```python
from build123d import *

# Parameters (mm, degrees)
SKETCH_1_W               = 38
SKETCH_1_H               = 12
EXTRUDE_1_DEPTH          = 1.6
EXTRUDE_START            = 1.6
SKETCH_1_3_W             = 38
SKETCH_1_3_H             = 1
SKETCH_1_3_W_2           = 1.5
SKETCH_1_3_H_2           = 12
EXTRUDE_2_DEPTH          = 1.5
EXTRUDE_START_2          = 3.1
EXTRUDE_3_DEPTH          = 8.4
SKETCH_2_4_W             = 2.1
SKETCH_2_4_H             = 1.5
EXTRUDE_5_DEPTH          = 3.1
CUT_EXTRUDE_1_DEPTH      = 22.850629282
FILLET_1_R               = 3
EXTRUDE_4_REACH          = 28.771
SKETCH_3_R               = 1.45
CUT_EXTRUDE_2_DEPTH      = 27.771253239
CUT_EXTRUDE_2_DEPTH_BACK = 27.771253239
SKETCH_3_3_R             = 1.7
SKETCH_3_3_W             = 6.5
SKETCH_3_3_H             = 1.2
SKETCH_3_3_W_2           = 3.4
SKETCH_3_3_H_2           = 3.1
FILLET_2_R               = 2.8
FILLET_3_R               = 2.5
FILLET_4_R               = 1
FILLET_5_R               = 0.3
FILLET_6_R               = 2


with BuildPart() as part:
    # 草图1 → 凸台-拉伸1 (new body)
    with BuildSketch(Plane(origin=(0, 0, 0), x_dir=(1, 0, 0), z_dir=(0, 1, 0))):
        Rectangle(SKETCH_1_W, SKETCH_1_H)
    extrude(amount=EXTRUDE_1_DEPTH)

    # 草图1<3> → 凸台-拉伸2 (add)
    with BuildSketch(Plane(origin=(0, 0, 0), x_dir=(1, 0, 0), z_dir=(0, 1, 0)).offset(EXTRUDE_START)):
        with Locations((0, 4)):
            Rectangle(SKETCH_1_3_W, SKETCH_1_3_H)
        Rectangle(SKETCH_1_3_W, SKETCH_1_3_H)
        with Locations((0, -4)):
            Rectangle(SKETCH_1_3_W, SKETCH_1_3_H)
        with Locations((-11.75, 0)):
            Rectangle(SKETCH_1_3_W_2, SKETCH_1_3_H_2)
        with Locations((11.75, 0)):
            Rectangle(SKETCH_1_3_W_2, SKETCH_1_3_H_2)
    extrude(amount=EXTRUDE_2_DEPTH)

    # 草图2 → 凸台-拉伸3 (add)
    with BuildSketch(Plane(origin=(0, 0, 0), x_dir=(1, 0, 0), z_dir=(0, 1, 0)).offset(EXTRUDE_START_2)):
        Polygon((-3.3, 9.3), (-5.4, 9.3), (-5.4, -2.4), (-7.5, -2.4), (-7.5, -9.4), (-5.5, -9.4), (-5.5, -2.8), (-3.3, -2.8), align=None)
        Polygon((5.4, 9.3), (3.3, 9.3), (3.3, -2.8), (5.5, -2.8), (5.5, -9.4), (7.5, -9.4), (7.5, -2.4), (5.4, -2.4), align=None)
    extrude(amount=-EXTRUDE_3_DEPTH)

    # 草图2<4> → 凸台-拉伸5 (add)
    with BuildSketch(Plane(origin=(0, 0, 0), x_dir=(1, 0, 0), z_dir=(0, 1, 0))):
        with Locations((-6.45, 5.25)):
            Rectangle(SKETCH_2_4_W, SKETCH_2_4_H)
        with Locations((6.45, 5.25)):
            Rectangle(SKETCH_2_4_W, SKETCH_2_4_H)
    extrude(amount=EXTRUDE_5_DEPTH)

    # 草图2<3> → 切除-拉伸1 (cut, through all)
    with BuildSketch(Plane(origin=(0, 0, 0), x_dir=(1, 0, 0), z_dir=(0, 1, 0))):
        Polygon((0, -9.4), (0, -2.8), (-3.3, -2.8), (-5.4, -2.8), (-5.5, -2.8), (-5.5, -9.4), align=None)
        Polygon((3.3, -2.8), (0, -2.8), (0, -9.4), (5.5, -9.4), (5.5, -2.8), (5.4, -2.8), align=None)
    extrude(amount=CUT_EXTRUDE_1_DEPTH, mode=Mode.SUBTRACT)

    # 圆角1
    # the kernel refuses this fillet: 3 mm, written as the material it adds along each edge
    with BuildSketch(Plane(origin=(5.4, 7.154544011, 2.4), x_dir=(1, 0, 0), z_dir=(0, -1, 0))) as fillet_1_piece_1_section:
        with BuildLine():
            CenterArc((3, -2.861817604), FILLET_1_R, 107.457603124, 72.542396876)
            Line((0, -2.861817604), (0, 0))
            Line((0, 0), (2.1, 0))
        make_face()
    fillet_1_piece_1 = extrude(amount=12.454544011, mode=Mode.PRIVATE)
    fillet_1_piece_1 = split(fillet_1_piece_1, bisect_by=Plane(origin=(6.297598678, 1.6, 1.686657362), z_dir=(0, -1, 0)), keep=Keep.TOP, mode=Mode.PRIVATE)
    add(fillet_1_piece_1)
    with BuildSketch(Plane(origin=(-5.4, 0, 2.4), x_dir=(0, 0, -1), z_dir=(0, -1, 0))) as fillet_1_piece_2:
        with BuildLine():
            CenterArc((2.861817604, -3), FILLET_1_R, 90, 72.542396876)
            Line((0, -2.1), (0, 0))
            Line((0, 0), (2.861817604, 0))
        make_face()
    extrude(amount=5.3)

    # 草图3 → 凸台-拉伸4 (add, up to next)
    with BuildSketch(Plane(origin=(-5.5, 0, 0), x_dir=(0, 0, -1), z_dir=(1, 0, 0)), mode=Mode.PRIVATE) as extrude_4_sk1:
        with Locations((-7, -2.5)):
            Circle(SKETCH_3_R)
    extrude_4_tool1 = extrude(extrude_4_sk1.sketch, amount=EXTRUDE_4_REACH, mode=Mode.PRIVATE) - part.part
    add(extrude_4_tool1.solids().sort_by_distance((-5.5, -2.5, 7))[0])

    # 草图3<3> → 切除-拉伸2 (cut, two sides: drawn at the far end of the back side and taken through both)
    with BuildSketch(Plane(origin=(-5.5, 0, 0), x_dir=(0, 0, -1), z_dir=(1, 0, 0)).offset(-CUT_EXTRUDE_2_DEPTH_BACK)):
        with Locations((5.58, -2.5)):
            Circle(SKETCH_3_3_R)
        with Locations((6.05, -4.7)):
            Rectangle(SKETCH_3_3_W, SKETCH_3_3_H)
        with Locations((-7.7, 1.55)):
            Rectangle(SKETCH_3_3_W_2, SKETCH_3_3_H_2)
    extrude(amount=CUT_EXTRUDE_2_DEPTH + CUT_EXTRUDE_2_DEPTH_BACK, mode=Mode.SUBTRACT)

    # 圆角2
    # the kernel refuses this fillet: 2.8 mm, written as the material it takes off along each edge
    with BuildSketch(Plane(origin=(-1.5, 0, 9.4), x_dir=(0, 0, -1), z_dir=(1, 0, 0)), Plane(origin=(-14.5, 0, 9.4), x_dir=(0, 0, -1), z_dir=(1, 0, 0))) as fillet_2_piece_1:
        with BuildLine():
            CenterArc((FILLET_2_R, -FILLET_2_R), FILLET_2_R, 90, 90)
            Line((0, -FILLET_2_R), (0, 0))
            Line((0, 0), (FILLET_2_R, 0))
        make_face()
    extrude(amount=16, mode=Mode.SUBTRACT)
    with BuildSketch(Plane(origin=(-1.5, -5.3, 9.4), x_dir=(0, 0, -1), z_dir=(1, 0, 0)), Plane(origin=(-14.5, -5.3, 9.4), x_dir=(0, 0, -1), z_dir=(1, 0, 0))) as fillet_2_piece_2:
        with BuildLine():
            CenterArc((FILLET_2_R, FILLET_2_R), FILLET_2_R, 180, 90)
            Line((0, FILLET_2_R), (0, 0))
            Line((0, 0), (FILLET_2_R, 0))
        make_face()
    extrude(amount=16, mode=Mode.SUBTRACT)

    # 圆角3
    fillet_3_edges = [part.edges().sort_by_distance(p)[0] for p in [
        (-4.35, 3.1, -9.3),
        (4.35, 3.1, -9.3),
    ]]
    fillet(fillet_3_edges, radius=FILLET_3_R)

    # 圆角4
    fillet_4_edges = [part.edges().sort_by_distance(p)[0] for p in [
        (-4.35, -4.1, -9.3),
        (4.35, -4.1, -9.3),
    ]]
    fillet(fillet_4_edges, radius=FILLET_4_R)

    # 圆角5
    fillet_5_edges = [part.edges().sort_by_distance(p)[0] for p in [
        (-4.35, -4.1, -5.005543735),
        (4.35, -4.1, -5.005543735),
        (-4.35, -4.1, -6.154456265),
        (4.35, -4.1, -6.154456265),
    ]]
    fillet(fillet_5_edges, radius=FILLET_5_R)

    # 圆角6
    # the kernel refuses this fillet: 2 mm, written as the material it adds along each edge
    with BuildSketch(Plane(origin=(5.4, 3.1, 2.4), x_dir=(0, 0, -1), z_dir=(0, -1, 0))) as fillet_6_piece_1:
        with BuildLine():
            CenterArc((2, 1.997498436), FILLET_6_R, 180, 87.134016017)
            Line((0, 1.997498436), (-0.04, 1.997498436))
            Line((-0.04, 1.997498436), (-0.04, 0))
            Line((-0.04, 0), (0, -0.04))
            ThreePointArc((0, -0.04), (0.95, -0.04), (1.898, -0.039949969))
            Line((1.898, -0.039949969), (1.9, 0))
        make_face()
    extrude(amount=6.493746089)
    with BuildSketch(Plane(origin=(-5.4, 3.1, 2.4), x_dir=(-1, 0, 0), z_dir=(0, -1, 0))) as fillet_6_piece_2:
        with BuildLine():
            CenterArc((1.997498436, 2), FILLET_6_R, 182.865983983, 87.134016017)
            Line((0, 1.9), (-0.039949969, 1.898))
            ThreePointArc((-0.039949969, 1.898), (-0.04, 0.95), (-0.04, 0))
            Line((-0.04, 0), (0, -0.04))
            Line((0, -0.04), (1.997498436, -0.04))
            Line((1.997498436, -0.04), (1.997498436, 0))
        make_face()
    extrude(amount=6.493746089)


solid = part.part
```
Source: CAD feature listing. Evaluate the final solid. Frame: model axes, mm. A direction names the side the tool comes from. Give positions to 0.01 mm unless a question says otherwise; leave off trailing zeros. Order: outer loops, then holes, each group sorted by start corner. A loop starts at its lowest first (then second) coordinate and runs counter-clockwise, first axis right, second up.
(1) Material intervals for line 1 along Z through (x, y) = (-4, -2.5); line 2 along X through (y, z) = (-0.5, -5.5); line 3 along X through (y, z) = (-4, 5.5), sorted ascending.
(2) Contact query for flat-ended pins moving along their axis: P1, Ø1, axis at x = -2.5, z = -2, coming from the -Y side; P2, Ø1.6, axis at x = -10, y = 1, coming from the +Z side; P3, Ø1.6, axis at x = 8.5, y = 2.5, coming from the -Z side. Output: stop coordinate, or through.
(3) Section query D-D (x = -13). Return the cut outline in (y, z).
(4) Access query for faces 1 (the face through (12.5, 2, 2)), 2 (the face through (-9, 2, -4.5)), 3 (the face through (-11, 2, 5)), 4 (the face through (4, -4.1, -8)). Directions: +Z, -Z, +X, -X, +Y, -Y. A direction counts if a zero-diameter tool reaches every point of the face in a straight line with its end or side. Return the directions, or none.
(5) Section query C-C (z = -7.75). Return the cut outline in (x, y), plus the area to 3 significant figures.
(6) Section query B-B (y = -4.5). Return the cut outline in (x, z), plus the area to 3 significant figures.
(7) Section query A-A (x = 1). Return the cut outline in (y, z).
(8) Pull-direction query (Z, two-part tool) for faces 5 (the face through (12.5, 2, 5)), 6 (the face through (-11, 2, -2)), 7 (the face through (-4, -5, -2.8)); classes: +Z half, -Z half, draft (parallel to the pull), parting line (faces both ways), or undercut.
Outcome:
1. line 1: z = -9.3 to -7.28, -3.88 to 2.8, 5.55 to 8.45
1. line 2: x = -5.4 to -3.3, 3.3 to 5.4
1. line 3: x = -7.5 to -5.5, 5.5 to 7.5
2. P1: stops at y = 0
2. P2: stops at z = 6
2. P3: stops at z = -4.5
3. outline: (0, -6) - (1.6, -6) - (1.6, -4.5) - (3.1, -4.5) - (3.1, -3.5) - (1.6, -3.5) - (1.6, -0.5) - (3.1, -0.5) - (3.1, 0.5) - (1.6, 0.5) - (1.6, 3.5) - (3.1, 3.5) - (3.1, 4.5) - (1.6, 4.5) - (1.6, 6) - (0, 6) - close
4. face 1: +X, +Y
4. face 2: -Z, +Y
4. face 3: +Z, +Y
4. face 4: -Z, +X, -X, -Y
5. outline: (-5.4, -4.1) - (-3.3, -4.1) - (-3.3, 2.91) - (-5.4, 2.91) - close; (3.3, -4.1) - (5.4, -4.1) - (5.4, 2.91) - (3.3, 2.91) - close
5. area: 29.5 mm2
6. outline: (-7.5, 2.4) arc R3 cw to (-5.4, -0.46) - (-5.4, -2.8) - (-3.3, -2.8) - (-3.3, 2.8) - (-5.5, 2.8) - (-5.5, 8.56) - (-7.5, 8.56) - close; (3.3, -2.8) - (5.4, -2.8) - (5.4, -0.46) arc R3 cw to (7.5, 2.4) - (7.5, 8.56) - (5.5, 8.56) - (5.5, 2.8) - (3.3, 2.8) - close
6. area: 51.4 mm2
7. outline: circle Ø2.9 at (-2.5, 7); (0, -6) - (1.6, -6) - (1.6, -4.5) - (3.1, -4.5) - (3.1, -3.5) - (1.6, -3.5) - (1.6, -0.5) - (3.1, -0.5) - (3.1, 0.5) - (1.6, 0.5) - (1.6, 2.8) - (0, 2.8) - close
8. face 5: draft
8. face 6: undercut
8. face 7: -Z half
